Here's how the part is built. I have some questions about the finished solid (model axes, mm). A direction names the side the tool comes from. Give positions to 0.01 mm unless a question says otherwise; leave off trailing zeros. Write each loop counter-clockwise with the first axis right and the second up, starting at its lowest first coordinate (ties: lowest second). Pieces come first, ordered by that corner, then holes. Notation, with made-up numbers: (10.5, 5) -> (50.5, 5) arc R22 cw to (50.5, 28) -> close; hole circle Ø2 at (48, 39). An arc over 180 degrees is marked (long way). Return JSON: item names as keys, results as strings.
Autodesk Inventor part; units mm, degrees
ref_plane "Work Plane1" through (124.725, 49.8, -24.875) normal (0, 1, 0) x (0, 0, 1)
ref_plane "YZ Plane" through (0, 0, 0) normal (1, 0, 0) x (0, 1, 0)
ref_plane "XZ Plane" through (0, 0, 0) normal (0, 1, 0) x (-1, 0, 0)
sketch "Sketch1" plane through (0, 0, 0) normal (0, 1, 0) x (-1, 0, 0)
  line L0 (-155.225, -15) -> (-155.225, 15)
  line L1 (-155.225, 15) -> (-147.725, 15)
  line L2 (-147.725, 15) -> (-147.725, -15)
  line L3 (-147.725, -15) -> (-155.225, -15)
  circle A0 centre (-171.5, -21.9) radius 1.875
  circle A1 centre (-127.7, 21.9) radius 1.875
  circle A2 centre (-127.7, -21.9) radius 1.875
  circle A3 centre (-171.5, 21.9) radius 1.875
  circle A4 centre (-135.2, 20.8) radius 2.0734
  circle A5 centre (-164, -20.8) radius 2.0734
  circle A6 centre (-135.2, -20.8) radius 2.0734
  circle A7 centre (-128.8, -14.4) radius 2.0734
  circle A8 centre (-128.8, 14.4) radius 2.0734
  circle A9 centre (-164, 20.8) radius 2.0734
  circle A10 centre (-170.4, -14.4) radius 2.0734
  circle A11 centre (-170.4, 14.4) radius 2.0734
  line L4 (-172.5, 24.875) -> (-126.7, 24.875)
  arc A12 (-172.5, 24.875) -> (-174.475, 22.9) centre (-172.5, 22.9) ccw
  line L5 (-174.475, -22.9) -> (-174.475, 22.9)
  arc A13 (-174.475, -22.9) -> (-172.5, -24.875) centre (-172.5, -22.9) ccw
  line L6 (-126.7, -24.875) -> (-172.5, -24.875)
  arc A14 (-126.7, -24.875) -> (-124.725, -22.9) centre (-126.7, -22.9) ccw
  line L7 (-124.725, 22.9) -> (-124.725, -22.9)
  arc A15 (-124.725, 22.9) -> (-126.7, 24.875) centre (-126.7, 22.9) ccw
  point P0 (0, 0)
ref_plane "Work Plane1" through (124.725, 49.8, -24.875) normal (0, 1, 0) x (0, 0, 1)
extrude "Extrusion1" add sketch "Sketch1" along normal blind 2 from surface at 49.8 contours A0 | A1 | A2 | A3 | L4 A15 L7 A14 L6 A13 L5 A12
sketch "Sketch2" plane through (126.7, 51.8, -24.875) normal (0, 1, 0) x (1, 0, 0)
  line L0 (28.525, -9.875) -> (21.025, -9.875)
  line L1 (28.525, -39.875) -> (28.525, -9.875)
  line L2 (21.025, -39.875) -> (28.525, -39.875)
  line L3 (21.025, -9.875) -> (21.025, -39.875)
  circle A0 centre (8.5, -45.675) radius 2.0734
  circle A1 centre (37.3, -4.075) radius 2.0734
  circle A2 centre (8.5, -4.075) radius 2.0734
  circle A3 centre (2.1, -10.475) radius 2.0734
  circle A4 centre (2.1, -39.275) radius 2.0734
  circle A5 centre (37.3, -45.675) radius 2.0734
  circle A6 centre (43.7, -10.475) radius 2.0734
  circle A7 centre (43.7, -39.275) radius 2.0734
  arc A8 (47.775, -1.975) -> (45.8, 0) centre (45.8, -1.975) ccw
  line L4 (0, 0) -> (45.8, 0)
  arc A9 (0, 0) -> (-1.975, -1.975) centre (0, -1.975) ccw
  line L5 (-1.975, -47.775) -> (-1.975, -1.975)
  arc A10 (-1.975, -47.775) -> (0, -49.75) centre (0, -47.775) ccw
  line L6 (45.8, -49.75) -> (0, -49.75)
  arc A11 (45.8, -49.75) -> (47.775, -47.775) centre (45.8, -47.775) ccw
  line L7 (47.775, -1.975) -> (47.775, -47.775)
  line L8 (16.025, -44.875) -> (33.525, -44.875)
  line L9 (33.525, -44.875) -> (33.525, -4.875)
  line L10 (33.525, -4.875) -> (16.025, -4.875)
  line L11 (16.025, -4.875) -> (16.025, -44.875)
  line L12 (45.8, 0) -> (50.05, 0)
  line L13 (50.05, 0) -> (50.05, -49.75)
  line L14 (50.05, -49.75) -> (45.8, -49.75)
  line L15 (45.8, -49.75) -> (45.8, 0)
  line L16 (50.05, -49.75) -> (47.925, -49.75)
  line L17 (47.925, -49.75) -> (47.925, 0)
  line L18 (47.925, 0) -> (50.05, 0)
  line L19 (50.05, 0) -> (50.05, -49.75)
  arc A12 (45.8, -49.875) -> (47.9, -47.775) centre (45.8, -47.775) ccw
  line L20 (45.8, -49.875) -> (0, -49.875)
  arc A13 (-2.1, -47.775) -> (0, -49.875) centre (0, -47.775) ccw
  line L21 (-2.1, -47.775) -> (-2.1, -1.975)
  arc A14 (0, 0.125) -> (-2.1, -1.975) centre (0, -1.975) ccw
  line L22 (0, 0.125) -> (45.8, 0.125)
  arc A15 (47.9, -1.975) -> (45.8, 0.125) centre (45.8, -1.975) ccw
  line L23 (47.9, -1.975) -> (47.9, -47.775)
  point P0 (-126.7, -24.875)
  point P1 (47.925, -49.75)
  point P2 (46.5137, -49.75)
  point P3 (46.5137, 0)
  dimension "d2" = 5
  dimension "d3" = 4.25
  dimension "d4" = 2.125
  dimension "d15" = 0.125
extrude "Extrusion2" cut sketch "Sketch2" against normal up to surface (2 mm away) contours L11 L10 L9 L8
extrude "Extrusion3" add sketch "Sketch2" against normal blind 2 contours A8 L12 A15 L23 A12 L14 A11 L7 | L12 L17 L14 A12 L23 A15 | L12 L13 L14 L17
extrude "Extrusion4" add sketch "Sketch2" against normal blind 49.8 from surface at -2 contours L12 L17 L14 A12 L23 A15 | L12 L13 L14 L17
fillet "Fillet1" radius 2 2 edges at (176.75, 25.9, 24.875) (176.75, 25.9, -24.875)
sketch "Sketch3" plane through (176.75, 51.8, 22.875) normal (1, 0, 0) x (0, 0, -1)
  line L0 (7.875, -21.425) -> (7.875, -28.925)
  line L1 (7.875, -28.925) -> (37.875, -28.925)
  line L2 (37.875, -28.925) -> (37.875, -21.425)
  line L3 (37.875, -21.425) -> (7.875, -21.425)
  line L4 (5.825, -9.7) -> (39.925, -9.7)
  line L5 (39.925, -44.1) -> (39.925, -9.7)
  line L6 (5.825, -44.1) -> (39.925, -44.1)
  line L7 (5.825, -9.7) -> (5.825, -44.1)
  line L8 (2.875, -16.425) -> (2.875, -33.925)
  line L9 (2.875, -33.925) -> (42.875, -33.925)
  line L10 (42.875, -33.925) -> (42.875, -16.425)
  line L11 (42.875, -16.425) -> (2.875, -16.425)
  point P0 (22.875, -51.8)
  dimension "d12" = 5
extrude "Extrusion5" cut sketch "Sketch3" against normal up to surface (2.15 mm away) contours L3 L2 L1 L0 | L11 L5 L9 L7 | L7 L9 L8 L11 | L11 L10 L9 L5
properties part number "Lens Light Cover"
1. Suppose I cut it at D-D, the plane z = -4.5. List the corners of the cut face in (x, y) for me (3 decimals).
Taken from the geometry:
{"outline": "(124.725, 49.8) -> (142.725, 49.8) -> (142.725, 51.8) -> (124.725, 51.8) -> close; (160.225, 49.8) -> (174.6, 49.8) -> (174.6, 35.375) -> (176.75, 35.375) -> (176.75, 51.8) -> (160.225, 51.8) -> close; (174.6, 0) -> (176.75, 0) -> (176.75, 17.875) -> (174.6, 17.875) -> close"}
2. If I drill on line 1 (Z direction, x = 164, y = 51.2) (3 decimals); line 2 (X direction, y = 50, z = -14) (3 decimals); line 3 (Z direction, x = 128, y = 51) (3 decimals), over which ranges is the centre line in solid material (lowest first)? Write a range as [from, to].
Taken from the geometry:
{"line 1": "z = [-24.875, -22.873], [-18.727, 18.727], [22.873, 24.875]", "line 2": "x = [124.725, 126.766], [130.834, 142.725], [160.225, 168.366], [172.434, 176.75]", "line 3": "z = [-24.875, -16.313], [-12.487, 12.487], [16.313, 24.875]"}
3. Suppose I cut it at B-B, the plane x = 135.2. List the corners of the cut face in (y, z) for me (3 decimals).
Taken from the geometry:
{"outline": "(49.8, -24.875) -> (51.8, -24.875) -> (51.8, -22.873) -> (49.8, -22.873) -> close; (49.8, -18.727) -> (51.8, -18.727) -> (51.8, 18.727) -> (49.8, 18.727) -> close; (49.8, 22.873) -> (51.8, 22.873) -> (51.8, 24.875) -> (49.8, 24.875) -> close"}
4. For pin 1 Ø1.1 at (x, y) = (176, 26) entering from -Z; pin 2 Ø5.5 at (x, z) = (128.8, 14.4) entering from -Y; pin 3 Ø1.7 at (x, z) = (175.5, 5.5) entering from -Y; pin 4 Ø13.5 at (y, z) = (24, -7.5) entering from -X, each with a flat end and sliding along its axis, tell me the tip position at first contact or that it passes through.
Taken from the geometry:
{"pin 1": "stops at z = -24.75", "pin 2": "stops at y = 49.8", "pin 3": "stops at y = 0", "pin 4": "stops at x = 174.6"}
5. If we mould it in two halves opening along Z, with no side actions, what happens to faces 1 (the face through (176, 0, 0)), 2 (the face through (151, 51, 20)), 3 (the face through (176.149, 25.537, -24.305))? For each: released by +Z, released by -Z, zero draft, split by the parting line, or undercut.
Taken from the geometry:
{"face 1": "zero draft", "face 2": "undercut", "face 3": "released by -Z"}
6. Suppose I cut it at C-C, the plane y = 30.5. List the corners of the cut face in (x, z) for me (3 decimals), and give its area (3 significant figures).
Taken from the geometry:
{"outline": "(173.214, -24.875) -> (174.75, -24.875) arc R2 ccw to (176.75, -22.875) -> (176.75, -20) -> (174.6, -20) -> (174.6, -22.9) arc R2.1 cw to start; (173.214, 24.875) arc R2.1 cw to (174.6, 22.9) -> (174.6, 20) -> (176.75, 20) -> (176.75, 22.875) arc R2 ccw to (174.75, 24.875) -> close", "area": "20.7 mm²"}
7. Which directions (+Z, -Z, +X, -X, +Y, -Y) give clear straight access to the entire face, cutting with the end or side of a thin tool? Please do faces 4 (the face through (176, 27, -20)), 5 (the face through (142.725, 51, 0)), 6 (the face through (174.21, 25.25, 24.12)), 7 (the face through (174, 37, -24.875)).
Taken from the geometry:
{"face 4": "+X, -X", "face 5": "+Y, -Y", "face 6": "-X, -Y", "face 7": "-Z, +X, -X, +Y, -Y"}
8. Suppose I cut it at A-A, the plane z = -14.4. List the corners of the cut face in (x, y) for me (3 decimals).
Taken from the geometry:
{"outline": "(124.725, 49.8) -> (126.727, 49.8) -> (126.727, 51.8) -> (124.725, 51.8) -> close; (130.873, 49.8) -> (142.725, 49.8) -> (142.725, 51.8) -> (130.873, 51.8) -> close; (160.225, 49.8) -> (168.327, 49.8) -> (168.327, 51.8) -> (160.225, 51.8) -> close; (172.473, 49.8) -> (174.6, 49.8) -> (174.6, 35.375) -> (176.75, 35.375) -> (176.75, 51.8) -> (172.473, 51.8) -> close; (174.6, 0) -> (176.75, 0) -> (176.75, 17.875) -> (174.6, 17.875) -> close"}
